Could you check a few things on this model? Use its own coordinates, in mm. Face numbers are marked on the shaded views. A direction names the side the tool comes from. Give positions to 0.01 mm unless a question says otherwise; leave off trailing zeros. Order: outer loops, then holes, each group sorted by start corner. A loop starts at its lowest first (then second) coordinate and runs counter-clockwise, first axis right, second up. Notation, with made-up numbers: (56, 27) - (80, 27) arc R30 ccw to (80, 56) - close; hole circle Ø1 at (-38, 68.5). An arc over 180 degrees is marked (long way). One line per question, with ' | ' between items. Start each with the question number.
1. If we mould it in two halves opening along X, with no side actions, what happens to the marked faces 1, 2 and 3? For each: released by +X, released by -X, zero draft, split by the parting line, or undercut.
2. Imagine slicing it at B-B (y = -11). Please give me the cut outline in (x, z).
3. Imagine slicing it at D-D (x = 22). Please give me the cut outline in (y, z).
4. Imagine slicing it at A-A (z = 10). Please give me the cut outline in (x, y).
5. Imagine slicing it at C-C (y = -19.75). Please give me the cut outline in (x, z), and give its area (3 significant figures).
6. For P1, Ø1, axis at x = -23, z = 9, coming from the -Y side; P2, Ø1.2, axis at x = -39, y = -17.5, coming from the -Z side; P3, Ø10, axis at y = 8, z = 10.5, coming from the +X side; P4, Ø6, axis at y = -4.5, z = 5, coming from the -X side, each with a flat end and sliding along its axis, tell me the tip position at first contact or that it passes through.
7. Which directions (+Z, -Z, +X, -X, +Y, -Y) give clear straight access to the entire face, cutting with the end or side of a thin tool? Please do the marked faces 4 and 5.
8. I need wall thicknesses on probe 1 along X at (y, z) = (-2, 11); probe 2 along Z at (x, y) = (37.2, -19.75); probe 3 along Z at (x, y) = (-37, -19). Which ranges of each line are inside material? Lowest first, please. Write a range as from..to.
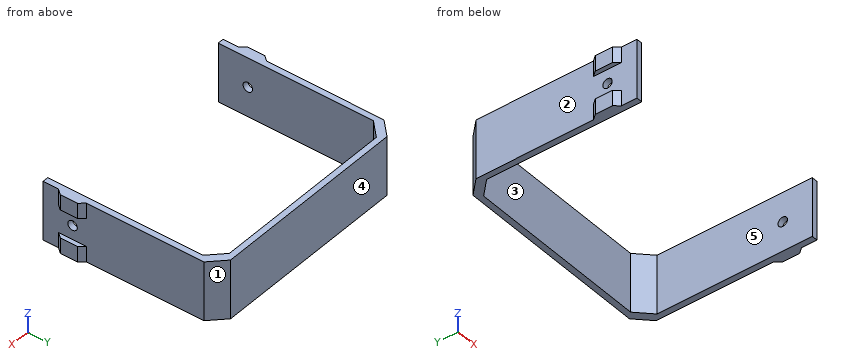
```python
from build123d import *

# Parameters (mm, degrees)
PAD_DEPTH       = 20
PAD001_DEPTH    = 20
SKETCH002_R     = 1.6
POCKET_DEPTH    = 3.5
SKETCH003_W     = 9.5
SKETCH003_H     = 9.5
POCKET001_DEPTH = 1.5
CHAMFER_SIZE    = 5


with BuildPart() as part:
    # Sketch → Pad (new body)
    with BuildSketch(Plane.XY):
        Polygon((-38.25, -29.75), (-38.25, 29.75), (38.25, 29.75), (38.25, -29.75), (36.25, -29.75), (36.25, 27.75), (-36.25, 27.75), (-36.25, -29.75), align=None)
    extrude(amount=PAD_DEPTH)

    # Sketch001 (on Face9 of Pad) → Pad001 (join)
    with BuildSketch(Plane(origin=(0, 0, 0), x_dir=(1, 0, 0), z_dir=(0, 0, -1))):
        Polygon((-38.25, 24.5), (-39.75, 22.7), (-39.75, 16.8), (-38.25, 15), align=None)
    pad001 = extrude(amount=-PAD001_DEPTH)

    # Sketch002 (on Face14 of Pad001) → Pocket (cut)
    with BuildSketch(Plane(origin=(-39.75, 0, 0), x_dir=(0, -1, 0), z_dir=(-1, 0, 0))):
        with Locations((19.75, 10)):
            Circle(SKETCH002_R)
    pocket = extrude(amount=-POCKET_DEPTH, mode=Mode.SUBTRACT)

    # Sketch003 (on Face14 of Pocket) → Pocket001 (cut)
    with BuildSketch(Plane(origin=(-39.75, 0, 0), x_dir=(0, -1, 0), z_dir=(-1, 0, 0))):
        with Locations((19.75, 10)):
            Rectangle(SKETCH003_W, SKETCH003_H)
    pocket001 = extrude(amount=-POCKET001_DEPTH, mode=Mode.SUBTRACT)

    # Mirrored: Pad001, Pocket, Pocket001 across YZ
    add(pad001.mirror(Plane.YZ))
    add(pocket.mirror(Plane.YZ), mode=Mode.SUBTRACT)
    add(pocket001.mirror(Plane.YZ), mode=Mode.SUBTRACT)

    # Chamfer
    chamfer_edges = [part.edges().sort_by_distance(p)[0] for p in [
        (36.25, 27.75, 10),
        (-36.25, 27.75, 10),
        (-38.25, 29.75, 10),
        (38.25, 29.75, 10),
    ]]
    chamfer(chamfer_edges, length=CHAMFER_SIZE)


solid = part.part
```
Results found:
1) face 1: released by +X | face 2: released by -X | face 3: undercut
2) outline: (-38.25, 0) - (-36.25, 0) - (-36.25, 20) - (-38.25, 20) - close; (36.25, 0) - (38.25, 0) - (38.25, 20) - (36.25, 20) - close
3) outline: (27.75, 0) - (29.75, 0) - (29.75, 20) - (27.75, 20) - close
4) outline: (-38.25, -29.75) - (-36.25, -29.75) - (-36.25, -21.35) - (-38.25, -21.35) - close; (-38.25, -18.15) - (-36.25, -18.15) - (-36.25, 22.75) - (-31.25, 27.75) - (31.25, 27.75) - (36.25, 22.75) - (36.25, -18.15) - (38.25, -18.15) - (38.25, 24.75) - (33.25, 29.75) - (-33.25, 29.75) - (-38.25, 24.75) - close; (36.25, -29.75) - (38.25, -29.75) - (38.25, -21.35) - (36.25, -21.35) - close
5) outline: (-39.75, 0) - (-36.25, 0) - (-36.25, 8.4) - (-38.25, 8.4) - (-38.25, 5.25) - (-39.75, 5.25) - close; (-39.75, 14.75) - (-38.25, 14.75) - (-38.25, 11.6) - (-36.25, 11.6) - (-36.25, 20) - (-39.75, 20) - close; (36.25, 0) - (39.75, 0) - (39.75, 5.25) - (38.25, 5.25) - (38.25, 8.4) - (36.25, 8.4) - close; (36.25, 11.6) - (38.25, 11.6) - (38.25, 14.75) - (39.75, 14.75) - (39.75, 20) - (36.25, 20) - close | area: 98.7 mm2
6) P1: stops at y = 27.75 | P2: stops at z = 0 | P3: stops at x = 38.25 | P4: stops at x = -38.25
7) face 4: +Z, -Z, +X, -X, +Y | face 5: +Z, -Z, -Y
8) probe 1: x = -38.25..-36.25, 36.25..38.25 | probe 2: z = 0..8.4, 11.6..20 | probe 3: z = 0..8.59, 11.41..20
